Can you work these out from the model? Positions are in its coordinate system, mm. Face numbers are marked on the shaded views. A direction names the side the tool comes from. Coordinates: 2 decimals unless noted, no trailing zeros. Write each loop counter-clockwise with the first axis right and the second up, starting at its lowest first coordinate (ties: lowest second). Pieces come first, ordered by that corner, then holes. Notation, with made-up numbers: (-8, -13) - (-1, -13) arc R9 cw to (-1, -9) - close; hole circle Ø1 at (36, -8.75). An arc over 180 degrees is marked (long way). Use one line per item in the form item = value. Start each with the question number.
(1) If we section it at D-D on y = 4: Please give me the cut outline in (x, z).
(2) On a 3-axis mill with a long thin cutter (end or side, diameter ignored), from which of +Z, -Z, +X, -X, +Y, -Y can I reach the whole of each face in a straight line? I mean the marked faces 4, 5, 6 and 7. Say none if no direction works.
(3) Thinking about a two-plate mould opening in X: for the marked faces 1, 2 and 3, which applies, pulls with the +X half, pulls with the -X half, needs draft (parallel to the pull), parting line crosses it, or undercut?
(4) If I drill on probe 1 along Z at (x, y) = (-5, 20.5); probe 2 along X at (y, z) = (2.25, 0.25); probe 3 along Z at (x, y) = (-3.5, 19), over which ranges is the centre line in solid material (lowest first)? Write a range as from..to.
(5) If we section it at C-C on z = 5.5: Please give me the cut outline in (x, y), then the cut area to 3 significant figures.
(6) If we section it at B-B on x = -1.5: Please give me the cut outline in (y, z), then the cut area to 3 significant figures.
(7) If we section it at A-A on y = 23: Please give me the cut outline in (x, z), then the cut area to 3 significant figures.
(8) For pin 1 Ø3 at (x, y) = (-3.5, 8) entering from -Z; pin 2 Ø4 at (x, y) = (-7.5, 10) entering from -Z; pin 3 Ø3 at (y, z) = (19, 8) entering from -X, each with a flat end and sliding along its axis, tell me the tip position at first contact or that it passes through.
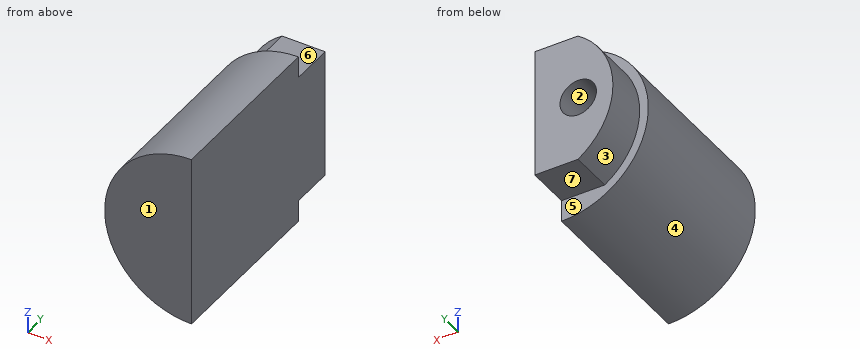
```python
from build123d import *

# Parameters (mm, degrees)
BOSS_EXTRUDE1_DEPTH   = 25
CUT_EXTRUDE1_DEPTH    = 5
M5_TAPPED_HOLE1_D     = 4.2
M5_TAPPED_HOLE1_DEPTH = 11.1381927
M5_TAPPED_HOLE1_TIP   = 1.2618073


with BuildPart() as part:
    # Sketch1 → Boss-Extrude1 (new body)
    with BuildSketch(Plane(origin=(0, 0, 0), x_dir=(1, 0, 0), z_dir=(0, 1, 0))):
        with BuildLine():
            Line((0, 10), (0, -10))
            ThreePointArc((0, -10), (-10, 0), (0, 10))
        make_face()
    extrude(amount=BOSS_EXTRUDE1_DEPTH)

    # Sketch18 → Cut-Extrude1 (cut)
    with BuildSketch(Plane(origin=(0, 25, 0), x_dir=(1, 0, 0), z_dir=(0, 1, 0))):
        with BuildLine():
            Line((0, 7.5), (0, 10))
            ThreePointArc((0, 10), (-10, 0), (0, -10))
            Line((0, -10), (0, -7.5))
            Line((0, -7.5), (-4.974937186, -7.5))
            ThreePointArc((-4.974937186, -7.5), (-9, 0), (-4.974937186, 7.5))
            Line((-4.974937186, 7.5), (0, 7.5))
        make_face()
    extrude(amount=-CUT_EXTRUDE1_DEPTH, mode=Mode.SUBTRACT)

    # M5 Tapped Hole1
    with Locations(Plane(origin=(0, 25, 0), x_dir=(1, 0, 0), z_dir=(0, 1, 0))):
        with Locations((-5, 0)):
            Hole(M5_TAPPED_HOLE1_D / 2, depth=M5_TAPPED_HOLE1_DEPTH)
            with Locations((0, 0, -(M5_TAPPED_HOLE1_DEPTH + M5_TAPPED_HOLE1_TIP / 2))):  # 118° drill point
                Cone(0, M5_TAPPED_HOLE1_D / 2, M5_TAPPED_HOLE1_TIP, mode=Mode.SUBTRACT)


solid = part.part
```
Reported:
q1.outline = (0, -10) - (0, 10) arc R10 ccw to start
q2.face_4 = -X, +Y, -Y
q2.face_5 = -X, +Y
q2.face_6 = +Z, +X, -X, +Y
q2.face_7 = -Z, +X, -X, +Y
q3.face_1 = needs draft
q3.face_2 = undercut
q3.face_3 = pulls with the -X half
q4.probe_1 = -7.48..-2.1, 2.1..7.48
q4.probe_2 = -10..0
q4.probe_3 = -9.37..-1.47, 1.47..9.37
q5.outline = (-8.35, 0) - (0, 0) - (0, 25) - (-7.12, 25) - (-7.12, 20) - (-8.35, 20) - close
q5.area = 203 mm2
q6.outline = (0, -9.89) - (20, -9.89) - (20, -7.5) - (25, -7.5) - (25, 7.5) - (20, 7.5) - (20, 9.89) - (0, 9.89) - close
q6.area = 470 mm2
q7.outline = (-4.97, -7.5) - (0, -7.5) - (0, 7.5) - (-4.97, 7.5) arc R9 ccw to start; hole circle Ø4.2 at (-5, 0)
q7.area = 103 mm2
q8.pin_1 = -9.8
q8.pin_2 = -8.35
q8.pin_3 = -7.6
